Geometry: final body of the model. Coordinates: model frame, mm. A direction names the side the tool comes from. Round coordinates to 2 decimals unless told otherwise and drop trailing zeros. Loops run counter-clockwise (first coordinate to the right, second up) from the corner with the lowest first, then second, coordinate; pieces in that order, holes last. Notation, with made-up numbers: (-2, 62) - (7, 62) arc R16 ccw to (7, 85) - close; hole circle Ø3 at (45, 27.25). An arc over 180 degrees is marked (long way). Answer as a JSON object with one key per item and string values. Group by question number.
Item 1: Draft query along Y for faces 4 (the face through (33.89, -25.01, 2.96)), 5 (the face through (34.421, 12.245, 3.972)), 6 (the face through (40, -15.5, 1.6)), 7 (the face through (-5, -5, 4)). Return one class per face: released by +Y, released by -Y, zero draft, split by the parting line, or undercut.
Item 2: Section B-B (x = -10). Return the cut outline in (y, z).
Item 3: Reachability of faces 1 (the face through (34.731, 2.855, 0.986)), 2 (the face through (33.41, 27.65, 3.97)), 3 (the face through (-6, 5, 4)) from +Z, -Z, +X, -X, +Y, -Y: full face, straight path, thin tool, end or side. Return the list, or none.
Item 4: Section C-C (z = 5). Count the separate pieces of the cut face and the enclosed holes in it, plus the area to 3 significant figures.
Item 5: Section A-A (z = 1). Return the cut outline in (x, y).
Item 6: First-contact query: pin 1 (1.2 mm diameter, centred on x = -8.5, z = 4.5, fed in from +Y); pin 2 (2 mm diameter, centred on y = -16, z = 0.5, fed in from -X); pin 3 (4 mm diameter, centred on x = 36.05, y = 22.65, fed in from -Z). Flat tips, straight axial feed; report the tip coordinate or a pass-through.
Item 7: Line query: line 1 (Y direction, x = 35, z = 3.7); line 2 (X direction, y = -24, z = 3.05); line 3 (Y direction, x = 18.5, z = 3.25). Output: solid intervals per line, ascending.
```python
from build123d import *

# Parameters (mm, degrees)
IZIM1_W                     = 80
IZIM1_H                     = 10
IZIM1_W_2                   = 10
IZIM1_H_2                   = 40
Y_KSEKLIK_EKSTR_ZYON1_DEPTH = 6
IZIM1_3_W                   = 70
IZIM1_3_H                   = 10
KES_EKSTR_ZYON1_DEPTH       = 2
IZIM4_R                     = 1.5
IZIM4_R_2                   = 1.65
Y_KSEKLIK_EKSTR_ZYON4_DEPTH = 4
IZIM4_3_R                   = 1.5
IZIM4_3_R_2                 = 1.65
KES_EKSTR_ZYON3_DEPTH       = 5
KES_EKSTR_ZYON5_START       = 6
IZIM4_6_R                   = 1.5
IZIM4_6_R_2                 = 1.65
KES_EKSTR_ZYON5_DEPTH       = 6


with BuildPart() as part:
    # Çizim1 → Yükseklik-Ekstrüzyon1 (new body)
    with BuildSketch(Plane.XY):
        Rectangle(IZIM1_W, IZIM1_H)
        with Locations((35, -8)):
            Rectangle(IZIM1_W_2, IZIM1_H_2)
    extrude(amount=Y_KSEKLIK_EKSTR_ZYON1_DEPTH)

    # Çizim1<3> → Kes-Ekstrüzyon1 (cut)
    with BuildSketch(Plane.XY):
        with Locations((-5, 0)):
            Rectangle(IZIM1_3_W, IZIM1_3_H)
    extrude(amount=KES_EKSTR_ZYON1_DEPTH, mode=Mode.SUBTRACT)

    # Çizim4 → Yükseklik-Ekstrüzyon4 (add)
    # profile 1 of 2: a face of its own
    with BuildSketch(Plane(origin=(0, 0, 2), x_dir=(-1, 0, 0), z_dir=(0, 0, -1))):
        with Locations((-35, -24)):
            Circle(IZIM4_R)
    # profile 2 of 2: a face of its own
    with BuildSketch(Plane(origin=(0, 0, 2), x_dir=(-1, 0, 0), z_dir=(0, 0, -1))):
        with BuildLine():
            Line((-29.73781884, 4.874886315), (-30.399690089, 22.862097513))
            ThreePointArc((-30.399690089, 22.862097513), (-33.487518923, 27.691929585), (-39.208988831, 27.335914357))
            Line((-39.208988831, 27.335914357), (-49.15078221, 20.618716695))
            ThreePointArc((-49.15078221, 20.618716695), (-51.725626297, 15.799448116), (-49.197080807, 10.955727499))
            Line((-49.197080807, 10.955727499), (-39.45690441, 4.237918054))
            ThreePointArc((-39.45690441, 4.237918054), (-34.486628982, 2.866804599), (-29.73781884, 4.874886315))
        make_face()
        with Locations((-36.045868913, 22.654336377)):
            Circle(IZIM4_R_2, mode=Mode.SUBTRACT)
        with Locations((-45.875693444, 15.771419141)):
            Circle(IZIM4_R_2, mode=Mode.SUBTRACT)
        with Locations((-35, 10.7)):
            Circle(IZIM4_R_2, mode=Mode.SUBTRACT)
    extrude(amount=-Y_KSEKLIK_EKSTR_ZYON4_DEPTH)

    # Çizim4<3> → Kes-Ekstrüzyon3 (cut, symmetric)
    with BuildSketch(Plane(origin=(0, 0, 2), x_dir=(-1, 0, 0), z_dir=(0, 0, -1))):
        with Locations(Location((-35, -24, 0), (0, 0, 180))):
            Circle(IZIM4_3_R)
        with Locations((-45.875693444, 15.771419141)):
            Circle(IZIM4_3_R_2)
        with Locations(Location((-35, 10.7, 0), (0, 0, 51.987720456))):
            Circle(IZIM4_3_R_2)
    extrude(amount=KES_EKSTR_ZYON3_DEPTH, both=True, mode=Mode.SUBTRACT)

    # Çizim4<6> → Kes-Ekstrüzyon5 (cut)
    # profile 1 of 2: a face of its own
    with BuildSketch(Plane(origin=(0, 0, 2), x_dir=(-1, 0, 0), z_dir=(0, 0, -1)).offset(KES_EKSTR_ZYON5_START)):
        with Locations(Location((-35, -24, 0), (0, 0, 180))):
            Circle(IZIM4_6_R)
    # profile 2 of 2: a face of its own
    with BuildSketch(Plane(origin=(0, 0, 2), x_dir=(-1, 0, 0), z_dir=(0, 0, -1)).offset(KES_EKSTR_ZYON5_START)):
        with BuildLine():
            Line((-29.73781884, 4.874886315), (-30.399690089, 22.862097513))
            ThreePointArc((-30.399690089, 22.862097513), (-33.487518923, 27.691929585), (-39.208988831, 27.335914357))
            Line((-39.208988831, 27.335914357), (-49.15078221, 20.618716695))
            ThreePointArc((-49.15078221, 20.618716695), (-51.725626297, 15.799448116), (-49.197080807, 10.955727499))
            Line((-49.197080807, 10.955727499), (-39.45690441, 4.237918054))
            ThreePointArc((-39.45690441, 4.237918054), (-34.486628982, 2.866804599), (-29.73781884, 4.874886315))
        make_face()
        with Locations((-36.045868913, 22.654336377)):
            Circle(IZIM4_6_R_2, mode=Mode.SUBTRACT)
        with Locations((-45.875693444, 15.771419141)):
            Circle(IZIM4_6_R_2, mode=Mode.SUBTRACT)
        with Locations((-35, 10.7)):
            Circle(IZIM4_6_R_2, mode=Mode.SUBTRACT)
    extrude(amount=-KES_EKSTR_ZYON5_DEPTH, mode=Mode.SUBTRACT)

    # Radyus2
    # a fillet whose section is not a circle: 40, 30 mm, written as the material it adds along each edge
    with BuildSketch(Plane(origin=(40, 4.612491628, 2), x_dir=(0, -1, 0), z_dir=(0, 0, 1))) as radyus2_piece_1:
        with BuildLine():
            Bezier((27.900120921, 0), (0, 0), (-5.027685175, 7.289659058), weights=[1, 0.885369562, 1])
            Line((-5.027685175, 7.289659058), (0, 0))
            Line((0, 0), (27.900120921, 0))
        make_face()
    extrude(amount=4)


solid = part.part
```
Values:
{
 "1": {"face 4": "undercut", "face 5": "undercut", "face 6": "zero draft", "face 7": "released by -Y"},
 "2": {"outline": "(-5, 2) - (5, 2) - (5, 6) - (-5, 6) - close"},
 "3": {"face 1": "-Z, +Y", "face 2": "+Z, -Z, +Y", "face 3": "+Z, -Z, -X, +Y"},
 "4": {"separate pieces": "1", "enclosed holes": "4", "area": "1,420 mm^2"},
 "5": {"outline": "(30, -28) - (40, -28) - (40, 4.61) - (39.46, 4.24) arc R7.85 cw to (30, 4.65) - close; hole circle Ø3 at (35, -24)"},
 "6": {"pin 1": "stops at y = 5", "pin 2": "stops at x = 30", "pin 3": "stops at z = 2"},
 "7": {"line 1": "y = -28 to -25.5, -22.5 to 9.05, 12.35 to 21.38, 23.93 to 28.21", "line 2": "x = 30 to 33.5, 36.5 to 40", "line 3": "y = -5 to 5"}
}
